```python
from build123d import *

# Parameters (mm, degrees)
F1_DEPTH = 12.7
F3_DEPTH = 75.184
F5_D     = 19.05


with BuildPart() as f1:
    # F0 (on Front) → F1 (new body)
    with BuildSketch(Plane.XZ):
        Polygon((-86.805733, 67.25759), (-86.805733, 0), (-14.163172, 0), (-51.245734, 67.25759), align=None)
    extrude(amount=F1_DEPTH)

    # F2 (on face) → F3 (join)
    with BuildSketch(Plane.XZ.offset(12.7)):
        Polygon((-54.981604, 56.942139), (-86.805733, 56.942139), (-86.805733, 0), (-23.58648, 0), align=None)
    extrude(amount=F3_DEPTH)

    # F5 (through all)
    with Locations(Plane(origin=(-18.087953, 0, -9.972817), x_dir=(0, 1, 0), z_dir=(0.875716, 0, 0.482827))):
        with Locations((-50.869141, 43.899961)):
            Hole(F5_D / 2)


solid = f1.part
```
Could you check a few things on this model? Use its own coordinates, in mm. A direction names the side the tool comes from. Give positions to 0.01 mm unless a question says otherwise; leave off trailing zeros. Write each loop counter-clockwise with the first axis right and the second up, starting at its lowest first coordinate (ties: lowest second). Pieces come first, ordered by that corner, then holes. Notation, with made-up numbers: (-17.5, 78) - (14.5, 78) arc R20 ccw to (14.5, 110) - close; hole circle Ø11 at (19.25, -3.75). An arc over 180 degrees is marked (long way). One line per item, written item: value. Start each with the question number.
Item 1: Imagine slicing it at C-C, the plane y = -8.5. List the corners of the cut face in (x, z) for me, and give its area (3 significant figures).
Item 2: Imagine slicing it at D-D, the plane y = -25. List the corners of the cut face in (x, z) for me.
Item 3: I'm going to push flat-ended pins straight in: pin 1 (5 mm diameter, centred on x = -43, y = -68, fed in from -Z); pin 2 (8 mm diameter, centred on y = -54, z = 52.5, fed in from +X); pin 3 (2 mm diameter, centred on x = -36, y = -30, fed in from +Z). Where does each tip first touch, or does it pass through?
Item 4: Imagine slicing it at B-B, the plane x = -28.5. List the corners of the cut face in (y, z) for me, and give its area (3 significant figures).
Item 5: Imagine slicing it at A-A, the plane z = 54. List the corners of the cut face in (x, y) for me, and give its area (3 significant figures).
Item 6: Please list where these lines run through material, in increasing order: line 1 (Y direction, x = -47.5, z = 15); line 2 (Y direction, x = -42.5, z = 18); line 3 (Z direction, x = -55, y = -82.5). Write a range as from..to.
Item 7: If we mould it in two halves opening along Y, with no side actions, what happens to faces 1 (the face through (-86.806, -43, 34)), 2 (the face through (-59, 0, 34)), 3 (the face through (-68.4, -49.6, 23.2))? For each: +Y half, -Y half, draft (parallel to the pull), parting line (faces both ways), or undercut.
Item 8: Which directions (+Z, -Z, +X, -X, +Y, -Y) give clear straight access to the entire face, cutting with the end or side of a thin tool? Please do faces 4 (the face through (-45, -12.7, 44)), 5 (the face through (-51, -43, 0)), 6 (the face through (-71, -50, 56.942)).
Geometry says:
1. outline: (-86.81, 0) - (-14.16, 0) - (-51.25, 67.26) - (-86.81, 67.26) - close
1. area: 3,640 mm^2
2. outline: (-86.81, 0) - (-23.59, 0) - (-54.98, 56.94) - (-86.81, 56.94) - close
3. pin 1: z = 0
3. pin 2: x = -50.33
3. pin 3: z = 24.33
4. outline: (-87.88, 0) - (0, 0) - (0, 26) - (-12.7, 26) - (-12.7, 8.91) - (-87.88, 8.91) - close
4. area: 1,000 mm^2
5. outline: (-86.81, -87.88) - (-53.36, -87.88) - (-53.36, -12.7) - (-43.94, -12.7) - (-43.94, 0) - (-86.81, 0) - close
5. area: 3,060 mm^2
6. line 1: -87.88..-56.29, -45.45..0
6. line 2: -87.88..-56.59, -45.15..0
6. line 3: 0..56.94
7. face 1: draft
7. face 2: +Y half
7. face 3: undercut
8. face 4: +Z, +X, -Y
8. face 5: -Z, +X, -X, +Y, -Y
8. face 6: +Z, +X, -X, -Y
